from build123d import *

# Parameters (mm, degrees)
SKETCH1_W           = 33.8
SKETCH1_H           = 6
BOSS_EXTRUDE1_DEPTH = 2
SKETCH2_W           = 2.5
SKETCH2_H           = 6
BOSS_EXTRUDE2_DEPTH = 25
SKETCH3_R           = 1.4
CUT_EXTRUDE1_DEPTH  = 44.364040402
FILLET1_R           = 3
SKETCH4_W           = 33.8
SKETCH4_H           = 2
BOSS_EXTRUDE3_DEPTH = 10
FILLET2_R           = 4


with BuildPart() as part:
    # Sketch1 → Boss-Extrude1 (new body)
    with BuildSketch(Plane.XY):
        Rectangle(SKETCH1_W, SKETCH1_H)
    extrude(amount=BOSS_EXTRUDE1_DEPTH)

    # Sketch2 → Boss-Extrude2 (add)
    with BuildSketch(Plane.XY.offset(2)):
        with Locations((-15.65, 0)):
            Rectangle(SKETCH2_W, SKETCH2_H)
        with Locations((15.65, 0)):
            Rectangle(SKETCH2_W, SKETCH2_H)
    extrude(amount=BOSS_EXTRUDE2_DEPTH)

    # Sketch3 → Cut-Extrude1 (cut, through all)
    with BuildSketch(Plane(origin=(16.9, 0, 0), x_dir=(0, 0, -1), z_dir=(1, 0, 0))):
        with Locations((-24.1, 0)):
            Circle(SKETCH3_R)
    extrude(amount=-CUT_EXTRUDE1_DEPTH, mode=Mode.SUBTRACT)

    # Fillet1
    fillet1_edges = [part.edges().sort_by_distance(p)[0] for p in [
        (-15.65, -3, 27),
        (15.65, -3, 27),
        (-15.65, 3, 27),
        (15.65, 3, 27),
    ]]
    fillet(fillet1_edges, radius=FILLET1_R - 0.0001)  # a hair under: the kernel refuses the full size

    # Sketch4 → Boss-Extrude3 (add)
    with BuildSketch(Plane(origin=(0, 3, 0), x_dir=(1, 0, 0), z_dir=(0, 1, 0))):
        with Locations((0, -1)):
            Rectangle(SKETCH4_W, SKETCH4_H)
    extrude(amount=BOSS_EXTRUDE3_DEPTH)

    # Fillet2
    fillet2_edges = [part.edges().sort_by_distance(p)[0] for p in [
        (14.4, 0, 2),
        (-14.4, 0, 2),
    ]]
    fillet(fillet2_edges, radius=FILLET2_R)


solid = part.part
Verification items for the finished model (mm, model axes). A direction names the side the tool comes from. Coordinates: 2 decimals unless noted, no trailing zeros. Order: outer loops, then holes, each group sorted by start corner. A loop starts at its lowest first (then second) coordinate and runs counter-clockwise, first axis right, second up. Notation, with made-up numbers: (-9.75, 0.5) -> (34.25, 0.5) arc R31 cw to (34.25, 39.5) -> close; hole circle Ø3 at (29, 21). An arc over 180 degrees is marked (long way). Put each result on its own line as item: value. Start each with the question number.
1. Go/stop test with flat-tipped pins: pin 1 Ø3 at (x, z) = (-13, 18) entering from +Y; pin 2 Ø2 at (y, z) = (0, 24.1) entering from +X; pin 3 Ø1 at (x, y) = (-11.5, 10) entering from +Z. Record where each tip stops, or that it passes through.
2. Access from +Z, -Z, +X, -X, +Y, -Y to the whole of each face (thin tool, end or side, straight path). Record for faces 1 (the flat face through (-15, 3, 13)), 2 (the flat face through (0, 5, 0)), 3 (the flat face through (0, 7, 2)), 4 (the flat face through (0, -3, 1)), 5 (the cylindrical face through (-13.259, 0.042, 3.203)).
3. Cross-section at B-B, the plane z = 24.5. Record the boundary of the cut face in (x, y), then the cut area to 3 significant figures.
4. Mould release check, pull along X, two halves, no side actions. Record for faces 6 (the cylindrical face through (13.259, 0.042, 3.203)), 7 (the cylindrical face through (15.67, -2.14, 26.1)), 8 (the flat face through (-16.9, 1, 11)): released by +X, released by -X, zero draft, split by the parting line, or undercut.
5. Cross-section at C-C, the plane y = 9. Record the boundary of the cut face in (x, z), then the cut area to 3 significant figures.
6. Cross-section at A-A, the plane z = 10.5. Record the boundary of the cut face in (x, y), then the cut area to 3 significant figures.
7. Cross-section at D-D, the plane x = -5.5. Record the boundary of the cut face in (y, z).
8. Material ranges on L1, parallel to Y at x = 15.8, z = 24.1; L2, parallel to X at y = -1.25, z = 18.75; L3, parallel to Z at x = 8.5, y = 6.5, recorded low to high. Write a range as [from, to].
Computed:
1. pin 1: y = 3
1. pin 2: through
1. pin 3: z = 2
2. face 1: +Z, +X, -X, +Y
2. face 2: -Z, +X, -X, +Y, -Y
2. face 3: +Z, +Y
2. face 4: +Z, -Z, +X, -X, -Y
2. face 5: +Z, +Y, -Y
3. outline: (-16.9, -2.96) -> (-14.4, -2.96) -> (-14.4, -1.34) -> (-16.9, -1.34) -> close; (-16.9, 1.34) -> (-14.4, 1.34) -> (-14.4, 2.96) -> (-16.9, 2.96) -> close; (14.4, -2.96) -> (16.9, -2.96) -> (16.9, -1.34) -> (14.4, -1.34) -> close; (14.4, 1.34) -> (16.9, 1.34) -> (16.9, 2.96) -> (14.4, 2.96) -> close
3. area: 16.2 mm2
4. face 6: undercut
4. face 7: zero draft
4. face 8: released by -X
5. outline: (-16.9, 0) -> (16.9, 0) -> (16.9, 2) -> (-16.9, 2) -> close
5. area: 67.6 mm2
6. outline: (-16.9, -3) -> (-14.4, -3) -> (-14.4, 3) -> (-16.9, 3) -> close; (14.4, -3) -> (16.9, -3) -> (16.9, 3) -> (14.4, 3) -> close
6. area: 30.0 mm2
7. outline: (-3, 0) -> (13, 0) -> (13, 2) -> (-3, 2) -> close
8. L1: [-3, -1.4], [1.4, 3]
8. L2: [-16.9, -14.4], [14.4, 16.9]
8. L3: [0, 2]
